Design review of the part built by this model. Coordinates are the model's own, in mm. A direction names the side the tool comes from. Coordinates: 2 decimals unless noted, no trailing zeros. Order: outer loops, then holes, each group sorted by start corner. A loop starts at its lowest first (then second) coordinate and runs counter-clockwise, first axis right, second up. Notation, with made-up numbers: (60, 42.5) -> (95, 42.5) arc R24 ccw to (95, 66.5) -> close; hole circle Ø4 at (80, 85.5). An arc over 180 degrees is marked (long way). Write item = value, one per line.
```python
from build123d import *

# Parameters (mm, degrees)
F1_DEPTH = 10
F2_W     = 29.5
F2_H     = 24
F3_DEPTH = 8
F5_DEPTH = 24
F6_R     = 1.5
F7_DEPTH = 30
F8_R     = 5


with BuildPart() as f1:
    # F0 (on Top) → F1 (new body)
    with BuildSketch(Plane.XY):
        Polygon((-28.717543, -14.298958), (-28.717543, -17.298958), (26.282457, -17.298958), (26.282457, 12.701042), (-28.717543, 12.701042), (-28.717543, 9.701042), (-6.217543, 9.701042), (-6.217543, -14.298958), align=None)
    extrude(amount=F1_DEPTH)

    # F2 (on face) → F3 (cut)
    with BuildSketch(Plane(origin=(0, 0, 0), x_dir=(1, 0, 0), z_dir=(0, 0, -1))):
        with Locations((8.532457, 2.298958)):
            Rectangle(F2_W, F2_H)
    extrude(amount=-F3_DEPTH, mode=Mode.SUBTRACT)

    # F4 (on face) → F5 (join)
    with BuildSketch(Plane.XZ.offset(-9.701042)):
        Polygon((23.282457, 2.5), (23.282457, 5.5), (20.282457, 5), (20.282457, 3), align=None)
    extrude(amount=F5_DEPTH)

    # F6 (on face) → F7 (cut)
    with BuildSketch(Plane(origin=(0, 12.701042, 0), x_dir=(-1, 0, 0), z_dir=(0, 1, 0))):
        with Locations((23.717543, 5)):
            Circle(F6_R)
    extrude(amount=-F7_DEPTH, mode=Mode.SUBTRACT)

    # F8
    f8_edges = [f1.edges().sort_by_distance(p)[0] for p in [
        (-28.717543, 11.201042, 0),
        (-28.717543, -15.798958, 0),
    ]]
    fillet(f8_edges, radius=F8_R)


solid = f1.part
```
(1) For faces 1 (the flat face through (-6.218, -2, 9)), 2 (the flat face through (-2, -17.299, 5)), 3 (the flat face through (21.761, -2.131, 2.754)), 4 (the flat face through (23.282, -2, 7)), list the 3-axis set-ups (+Z, -Z, +X, -X, +Y, -Y) from which the entire face can be reached by the end or side of a thin tool; tool diameter is ignored.
Report:
face_1 = +Z, -Z, -X
face_2 = +Z, -Z, +X, -X, -Y
face_3 = -Z, -X
face_4 = -X
(2) We need section B-B (y = -4.5). Write out the cut boundary in (x, z).
Report:
outline = (-6.22, 8) -> (23.28, 8) -> (23.28, 5.5) -> (20.28, 5) -> (20.28, 3) -> (23.28, 2.5) -> (23.28, 0) -> (26.28, 0) -> (26.28, 10) -> (-6.22, 10) -> close
(3) We need section C-C (x = 15.5). Write out the cut boundary in (y, z), and give its area (3 significant figures).
Report:
outline = (-17.3, 0) -> (-14.3, 0) -> (-14.3, 8) -> (9.7, 8) -> (9.7, 0) -> (12.7, 0) -> (12.7, 10) -> (-17.3, 10) -> close
area = 108 mm²
(4) For L1, parallel to Y at x = -4, z = 4; L2, parallel to X at y = -2.75, z = 1.75; L3, parallel to Z at x = 0.5, y = -6.5, list the stretches that pass through material, from the lowest coordinate up.
Report:
L1 = -17.3 to -14.3, 9.7 to 12.7
L2 = 23.28 to 26.28
L3 = 8 to 10
(5) Insertion check: pin 1 (1.6 mm diameter, centred on y = -5, z = 9, fed in from -X); pin 2 (12 mm diameter, centred on x = 13, y = -6.5, fed in from -Z); pin 3 (1.2 mm diameter, centred on y = 3, z = 1, fed in from -X). Each pin has a flat end and moves straight along its axis. Give the tip position at first contact, or say it passes through.
Report:
pin_1 = -6.22
pin_2 = 8
pin_3 = 23.28
(6) We need section A-A (x = -15). Write out the cut boundary in (y, z), and give its area (3 significant figures).
Report:
outline = (-17.3, 0) -> (-14.3, 0) -> (-14.3, 10) -> (-17.3, 10) -> close; (9.7, 0) -> (12.7, 0) -> (12.7, 10) -> (9.7, 10) -> close
area = 60.0 mm²
(7) The part is to be moulded in two halves that separate along X. For faces 5 (the cylindrical face through (-25.15, 11.22, 5.45)), 6 (the flat face through (5, -2, 10)), 7 (the flat face through (20.282, -2, 4)), say which applies: released by +X, released by -X, zero draft, split by the parting line, or undercut.
Report:
face_5 = undercut
face_6 = zero draft
face_7 = released by -X
